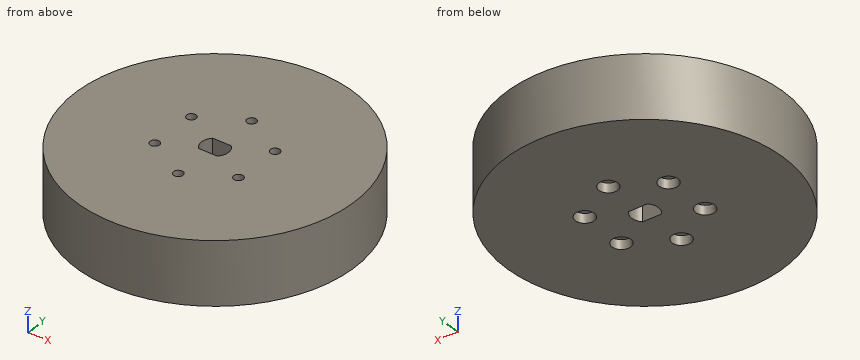
from build123d import *

# Parameters (mm, degrees)
SKETCH1_R           = 44
SKETCH1_R_2         = 4.25
BOSS_EXTRUDE1_DEPTH = 20
SKETCH2_R           = 1.5
CUT_EXTRUDE1_DEPTH  = 114.02795241
SKETCH2_3_R         = 3
CUT_EXTRUDE2_DEPTH  = 3
CIRPATTERN1_COUNT   = 6


with BuildPart() as part:
    # Sketch1 → Boss-Extrude1 (new body)
    # profile 1 of 3: a face of its own
    with BuildSketch(Plane.XY):
        with Locations((-42.570496177, 25.863203603)):
            Circle(SKETCH1_R)
        with Locations((-42.570496177, 25.863203603)):
            Circle(SKETCH1_R_2, mode=Mode.SUBTRACT)
    # profile 2 of 3: a face of its own
    with BuildSketch(Plane.XY):
        with BuildLine():
            ThreePointArc((-39.565292357, 28.868407423), (-42.570496177, 30.113203603), (-45.575699997, 28.868407423))
            Line((-45.575699997, 28.868407423), (-39.565292357, 28.868407423))
        make_face()
    # profile 3 of 3: a face of its own
    with BuildSketch(Plane.XY):
        with BuildLine():
            ThreePointArc((-45.575699997, 22.857999783), (-42.570496177, 21.613203603), (-39.565292357, 22.857999783))
            Line((-39.565292357, 22.857999783), (-45.575699997, 22.857999783))
        make_face()
    extrude(amount=BOSS_EXTRUDE1_DEPTH)

    # Sketch2 → Cut-Extrude1 (cut, through all)
    with BuildSketch(Plane(origin=(0, 0, 0), x_dir=(-1, 0, 0), z_dir=(0, 0, -1))):
        with Locations((42.570496177, 41.363203603)):
            Circle(SKETCH2_R)
    cut_extrude1 = extrude(amount=-CUT_EXTRUDE1_DEPTH, mode=Mode.SUBTRACT)

    # Sketch2_3 → Cut-Extrude2 (cut)
    with BuildSketch(Plane(origin=(0, 0, 0), x_dir=(-1, 0, 0), z_dir=(0, 0, -1))):
        with Locations((42.570496177, 41.363203603)):
            Circle(SKETCH2_3_R)
    cut_extrude2 = extrude(amount=-CUT_EXTRUDE2_DEPTH, mode=Mode.SUBTRACT)

    # CirPattern1: Cut-Extrude1, Cut-Extrude2 ×6 about axis
    cirpattern1_axis = Axis((-42.570496177, 25.863203603, 0), (0, 0, 1))
    add([cut_extrude1.rotate(cirpattern1_axis, i * 360 / CIRPATTERN1_COUNT) for i in range(1, CIRPATTERN1_COUNT)], mode=Mode.SUBTRACT)
    add([cut_extrude2.rotate(cirpattern1_axis, i * 360 / CIRPATTERN1_COUNT) for i in range(1, CIRPATTERN1_COUNT)], mode=Mode.SUBTRACT)


solid = part.part
The listing builds one solid part. Answer for the finished solid, in the listing's coordinates (mm). Coordinates: 2 decimals unless noted, no trailing zeros. Write each loop counter-clockwise with the first axis right and the second up, starting at its lowest first coordinate (ties: lowest second). Pieces come first, ordered by that corner, then holes. Notation, with made-up numbers: M 23.5,-5.75 L 51.5,-5.75 A9 ccw 51.5,8.25 Z; hole C -23.75,88.5 d8. An arc over 180 degrees is marked long. Put each result on its own line as item: value. Start each with the question number.
1. A cutting plane is placed at D-D on x = -68.5. Write down the section's boundary in (y, z), then the cut area to 3 significant figures.
2. Consider line 1 (Y direction, x = -54, z = 1.75); line 2 (Y direction, x = -56, z = 12.25); line 3 (Y direction, x = -46.5, z = 17.5). Determine where each line is inside the solid, lowest interval first. Write a range as from..to.
3. A cutting plane is placed at C-C on x = -34.5. Write down the section's boundary in (y, z).
4. A cutting plane is placed at A-A on y = 24.5. Write down the section's boundary in (x, z).
5. Flat-ended cylindrical pins translate along their axes: P1, Ø4, axis at x = -58.5, z = 15.5, coming from the -Y side; P2, Ø2, axis at x = -67, z = 4.5, coming from the +Y side; P3, Ø3, axis at x = -46.5, z = 11, coming from the -Y side; P4, Ø2.5, axis at x = -42.57, y = 10.36, coming from the +Z side. Find the tip coordinate at first contact, or state that the pin passes through.
6. A cutting plane is placed at B-B on z = 10.5. Write down the section's boundary in (x, y), then the cut area to 3 significant figures.
Resolved:
1. outline: M -9.68,0 L 61.41,0 L 61.41,20 L -9.68,20 Z
1. area: 1,420 mm2
2. line 1: y = -16.63..15.87, 20.35..31.37, 35.85..68.35
2. line 2: y = -16.04..16.61, 19.61..32.11, 35.11..67.76
2. line 3: y = -17.96..24.24, 27.48..69.69
3. outline: M -17.39,0 L 69.12,0 L 69.12,20 L -17.39,20 Z
4. outline: M -86.55,0 L -46.6,0 L -46.6,20 L -86.55,20 Z; M -38.55,0 L 1.41,0 L 1.41,20 L -38.55,20 Z
5. P1: stops at y = -15.87
5. P2: stops at y = 63.11
5. P3: stops at y = -18.07
5. P4: passes through
6. outline: C -42.57,25.86 d88; hole C -55.99,18.11 d3; hole C -55.99,33.61 d3; hole M -45.58,22.86 L -39.57,22.86 A4.25 ccw -39.57,28.87 L -45.58,28.87 A4.25 ccw Z; hole C -42.57,10.36 d3; hole C -42.57,41.36 d3; hole C -29.15,18.11 d3; hole C -29.15,33.61 d3
6. area: 5,990 mm2
